Build history of the part. All positions in model axes, mm. Face numbers are marked on the shaded views. A direction names the side the tool comes from. Round coordinates to 2 decimals unless told otherwise and drop trailing zeros. Loops run counter-clockwise (first coordinate to the right, second up) from the corner with the lowest first, then second, coordinate; pieces in that order, holes last. Notation, with made-up numbers: (77.5, 81.25) - (81.5, 81.25) arc R21 cw to (81.5, 115.25) - close; hole circle Ø11 at (68, 4.5). An arc over 180 degrees is marked (long way). Use a Markdown table: item, result.
from build123d import *

# Parameters (mm, degrees)
ESQUISSE1_W                = 50
ESQUISSE1_H                = 18
BOSS_EXTRU_1_DEPTH         = 3
ESQUISSE2_W                = 10
ESQUISSE2_H                = 3
ENL_V_MAT_EXTRU_1_DEPTH    = 3
R_P_TITION_LIN_AIRE1_COUNT = 2
R_P_TITION_LIN_AIRE1_PITCH = 20
ESQUISSE3_W                = 3
ESQUISSE3_H                = 10
ENL_V_MAT_EXTRU_2_DEPTH    = 3


with BuildPart() as part:
    # Esquisse1 → Boss.-Extru.1 (new body)
    with BuildSketch(Plane.XY):
        with Locations((25, -9)):
            Rectangle(ESQUISSE1_W, ESQUISSE1_H)
    extrude(amount=BOSS_EXTRU_1_DEPTH)

    # Esquisse2 → Enlèv. mat.-Extru.1 (cut)
    with BuildSketch(Plane.XY.offset(3)):
        with Locations((35, -16.5)):
            Rectangle(ESQUISSE2_W, ESQUISSE2_H)
    enl_v_mat_extru_1 = extrude(amount=-ENL_V_MAT_EXTRU_1_DEPTH, mode=Mode.SUBTRACT)

    # Répétition linéaire1: Enlèv. mat.-Extru.1 ×2
    with Locations(*[(-i * R_P_TITION_LIN_AIRE1_PITCH, 0, 0) for i in range(1, R_P_TITION_LIN_AIRE1_COUNT)]):
        add(enl_v_mat_extru_1, mode=Mode.SUBTRACT)

    # Esquisse3 → Enlèv. mat.-Extru.2 (cut)
    with BuildSketch(Plane.XY.offset(3)):
        with Locations((1.5, -5)):
            Rectangle(ESQUISSE3_W, ESQUISSE3_H)
    extrude(amount=-ENL_V_MAT_EXTRU_2_DEPTH, mode=Mode.SUBTRACT)


solid = part.part
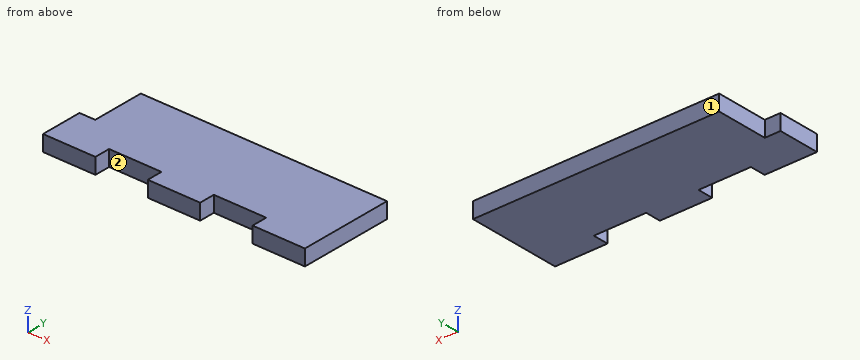
Q1. Probe line 1 (X direction, y = -15.5, z = 1.5); line 2 (Y direction, x = 33.5, z = 1.8); line 3 (X direction, y = -3.25, z = 2.45). List the from-to ranges inside material, lowest first.
Results found:
| item | result |
|---|---|
| line 1 | x = 0 to 10, 20 to 30, 40 to 50 |
| line 2 | y = -15 to 0 |
| line 3 | x = 3 to 50 |
Q2. Cut at A-A, the plane z = 2.35. List the corners of the cut face in (x, y), plus the area to 3 significant figures.
Results found:
| item | result |
|---|---|
| outline | (0, -18) - (10, -18) - (10, -15) - (20, -15) - (20, -18) - (30, -18) - (30, -15) - (40, -15) - (40, -18) - (50, -18) - (50, 0) - (3, 0) - (3, -10) - (0, -10) - close |
| area | 810 mm2 |
Q3. Cut at B-B, the plane x = 19.5. List the corners of the cut face in (y, z), plus the area to 3 significant figures.
Results found:
| item | result |
|---|---|
| outline | (-15, 0) - (0, 0) - (0, 3) - (-15, 3) - close |
| area | 45.0 mm2 |
Q4. Drop flat-ended pins along their axis: pin 1 (0.9 mm diameter, centred on x = 33, z = 1.5, fed in from -Y); pin 2 (0.9 mm diameter, centred on y = -3.5, z = 1, fed in from -X). Give the stop position or say it passes through.
Results found:
| item | result |
|---|---|
| pin 1 | stops at y = -15 |
| pin 2 | stops at x = 3 |
Q5. Which spindle directions (+Z, -Z, +X, -X, +Y, -Y) get a long thin tool onto all of the face, cutting with end or side? Do the marked faces 1 and 2. Say none if no direction does.
Results found:
| item | result |
|---|---|
| face 1 | +Z, -Z, +X, -X, +Y |
| face 2 | +Z, -Z, -Y |
Q6. Cut at C-C, the plane y = -6. List the corners of the cut face in (x, z), plus the area to 3 significant figures.
Results found:
| item | result |
|---|---|
| outline | (3, 0) - (50, 0) - (50, 3) - (3, 3) - close |
| area | 141 mm2 |
